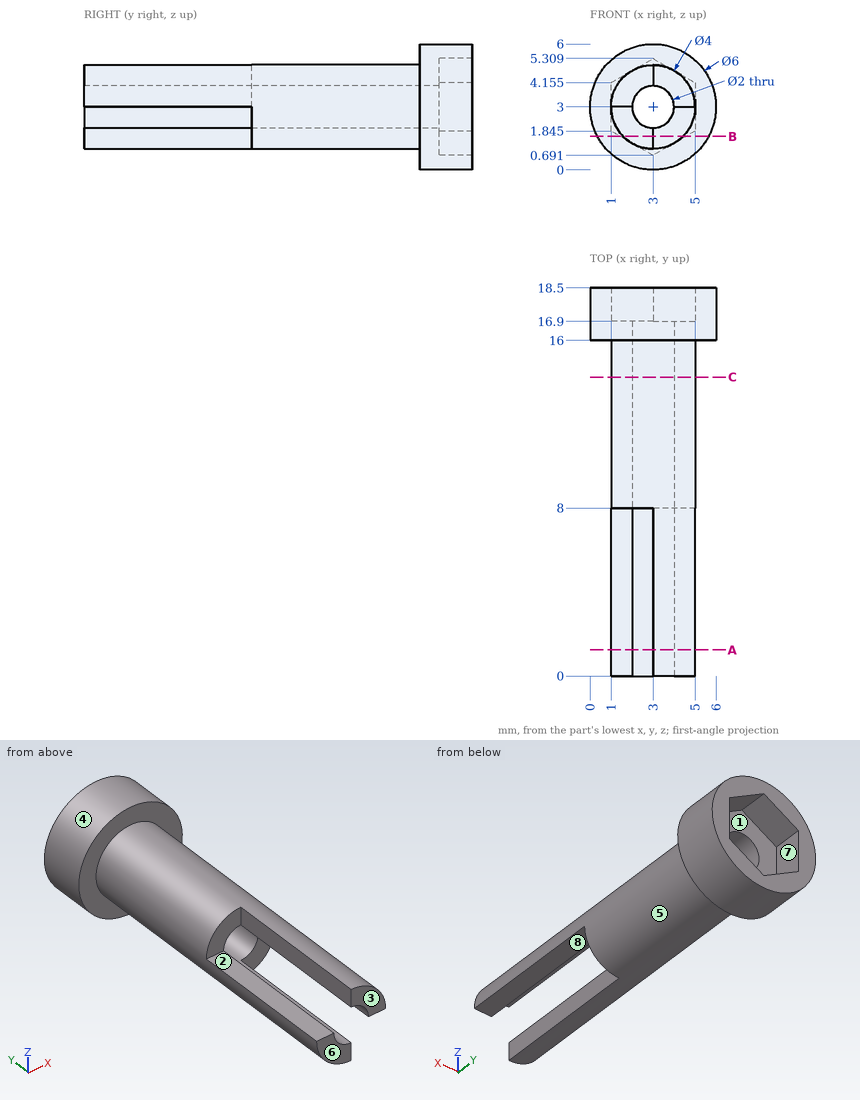
For this review, use the dimensioned drawing (mm, ordinates from the lowest corner) and the shaded views. A direction names the side the tool comes from. Give positions to 0.01 mm unless a question says otherwise; leave off trailing zeros. Write each loop counter-clockwise with the first axis right and the second up, starting at its lowest first coordinate (ties: lowest second). Pieces come first, ordered by that corner, then holes.
(1) Tool access review of the marked faces 1, 2, 3, 4 and 5: name each direction out of +Z, -Z, +X, -X, +Y, -Y from which nothing blocks a thin tool from reaching the whole face with its end or side.
(2) To check wall thickness, follow L1, parallel to Z at x = 3, y = 10.5; L2, parallel to Y at x = 2.65, z = 1.55. State the ranges of each line that lie inside material, in increasing order.
(3) Consider section B-B, the plane z = 1.6. Give the boundary of the cut face in (x, y) (1 decimal), and give its area (3 significant figures).
(4) Consider section C-C, the plane y = 14.25. Give the boundary of the cut face in (x, z).
(5) For P1, Ø1, axis at y = 2.5, z = 5, coming from the -X side; P2, Ø1, axis at x = 2.5, y = 4, coming from the -Z side; P3, Ø0.6, axis at x = 2, z = 4, coming from the -Y side, all flat-tipped, find the tip position at first contact; note any pin that passes through.
(6) The part is to be moulded in two halves that separate along Z. For the marked faces 6, 7 and 8, say which applies: released by +Z, released by -Z, zero draft, split by the parting line, or undercut.
(7) Consider section A-A, the plane y = 1.25. Give the boundary of the cut face in (x, z).
Returned:
1. face 1: +Y
1. face 2: +Z, -X, -Y
1. face 3: +Z, -Z, +X, -X, -Y
1. face 4: +Y, -Y
1. face 5: -Y
2. L1: z = 1 to 2, 4 to 5
2. L2: y = 0 to 16.9
3. outline: (0.3, 16) - (1.6, 16) - (1.6, 0) - (3, 0) - (3, 8) - (4.4, 8) - (4.4, 16) - (5.7, 16) - (5.7, 18.5) - (4.6, 18.5) - (4.6, 16.9) - (1.4, 16.9) - (1.4, 18.5) - (0.3, 18.5) - close
3. area: 42.5 mm2
4. outline: circle Ø4 at (3, 3); hole circle Ø2 at (3, 3)
5. P1: stops at x = 3
5. P2: stops at z = 1
5. P3: stops at y = 8
6. face 6: zero draft
6. face 7: undercut
6. face 8: released by -Z
7. outline: (1, 3) arc R2 ccw to (3, 1) - (3, 2) arc R1 cw to (2, 3) - close; (3, 4) arc R1 cw to (4, 3) - (5, 3) arc R2 ccw to (3, 5) - close
